```python
from build123d import *

# Parameters (mm, degrees)
V10_IMU_CANDIDATE18X20_START           = 38
SKETCH_2_W                             = 18
SKETCH_2_H                             = 20
V10_IMU_CANDIDATE18X20_DEPTH           = 1.6
V10_IMU_PACKAGE_START                  = 39.6
SKETCH_3_W                             = 6
SKETCH_3_H                             = 6
V10_IMU_PACKAGE_DEPTH                  = 1.4
SKETCH_4_R                             = 1.3
V10_IMU_DIAGONAL_CANDIDATE_HOLES_DEPTH = 1.6


with BuildPart() as part:
    # 草图2 → V10_IMU_candidate18x20 (new body)
    with BuildSketch(Plane.XY.offset(V10_IMU_CANDIDATE18X20_START)):
        with Locations((-65, -60)):
            Rectangle(SKETCH_2_W, SKETCH_2_H)
    extrude(amount=V10_IMU_CANDIDATE18X20_DEPTH)

    # 草图3 → V10_IMU_package (add)
    with BuildSketch(Plane.XY.offset(V10_IMU_PACKAGE_START)):
        with Locations((-65, -60)):
            Rectangle(SKETCH_3_W, SKETCH_3_H)
    extrude(amount=V10_IMU_PACKAGE_DEPTH)

    # 草图4 → V10_IMU_diagonal_candidate_holes (cut)
    with BuildSketch(Plane.XY.offset(39.6)):
        with Locations((-70, -66)):
            Circle(SKETCH_4_R)
        with Locations((-60, -54)):
            Circle(SKETCH_4_R)
    extrude(amount=-V10_IMU_DIAGONAL_CANDIDATE_HOLES_DEPTH, mode=Mode.SUBTRACT)


solid = part.part
```
Geometry check sheet. Reference: the model listing, model coordinates, mm. A direction names the side the tool comes from. Give positions to 0.01 mm unless a question says otherwise; leave off trailing zeros. Loops run counter-clockwise (first coordinate to the right, second up) from the corner with the lowest first, then second, coordinate; pieces in that order, holes last. Notation, with made-up numbers: (89, 4.5) - (148, 4.5) arc R18 cw to (148, 24.5) - close; hole circle Ø1 at (60.25, -34.75). An arc over 180 degrees is marked (long way). Use CSV: the item, a comma, the result in double quotes. Start each with the question number.
Q1. Scan lines: probe 1 along Y at (x, z) = (-60, 38.8); probe 2 along X at (y, z) = (-66, 38.6); probe 3 along Z at (x, y) = (-70.5, -64.75). Record each from-to range of solid material in increasing order. Write a range as from..to.
Q2. Section check B-B, the plane y = -66. Record the cut outline in (x, z).
Q3. Access from +Z, -Z, +X, -X, +Y, -Y to the whole of each face (thin tool, end or side, straight path). Record for faces 1 (the face through (-62, -60, 40)), 2 (the face through (-68, -60, 40)), 3 (the face through (-65, -63, 40)).
Q4. Release check for a two-part mould opening along X. For faces 4 (the face through (-65, -57, 40)), 5 (the face through (-74, -60, 39)), 6 (the face through (-59.301, -52.904, 38.811)) record: +X half, -X half, draft (parallel to the pull), parting line (faces both ways), or undercut.
Q5. Section check A-A, the plane x = -60. Record the cut outline in (y, z), and give its area (3 significant figures).
Q6. Section check C-C, the plane z = 38.7. Record the cut outline in (x, y), and give its area (3 significant figures).
Q7. Section check D-D, the plane y = -60.75. Record the cut outline in (x, z), and give its area (3 significant figures).
Q8. Go/stop test with flat-tipped pins: pin 1 Ø5 at (x, y) = (-71, -63) entering from +Z; pin 2 Ø1.5 at (y, z) = (-60, 40.5) entering from +X; pin 3 Ø0.7 at (y, z) = (-61, 40.5) entering from -X. Record where each tip stops, or that it passes through.
Findings below:
1,probe 1,"y = -70..-55.3, -52.7..-50"
1,probe 2,"x = -74..-71.3, -68.7..-56"
1,probe 3,"z = 38..39.6"
2,outline,"(-74, 38) - (-71.3, 38) - (-71.3, 39.6) - (-74, 39.6) - close; (-68.7, 38) - (-56, 38) - (-56, 39.6) - (-68.7, 39.6) - close"
3,face 1,"+Z, +X, +Y, -Y"
3,face 2,"+Z, -X, +Y, -Y"
3,face 3,"+Z, +X, -X, -Y"
4,face 4,"draft"
4,face 5,"-X half"
4,face 6,"undercut"
5,outline,"(-70, 38) - (-55.3, 38) - (-55.3, 39.6) - (-70, 39.6) - close; (-52.7, 38) - (-50, 38) - (-50, 39.6) - (-52.7, 39.6) - close"
5,area,"27.8 mm^2"
6,outline,"(-74, -70) - (-56, -70) - (-56, -50) - (-74, -50) - close; hole circle Ø2.6 at (-70, -66); hole circle Ø2.6 at (-60, -54)"
6,area,"349 mm^2"
7,outline,"(-74, 38) - (-56, 38) - (-56, 39.6) - (-62, 39.6) - (-62, 41) - (-68, 41) - (-68, 39.6) - (-74, 39.6) - close"
7,area,"37.2 mm^2"
8,pin 1,"stops at z = 39.6"
8,pin 2,"stops at x = -62"
8,pin 3,"stops at x = -68"
